Here's how the part is built. I have some questions about the finished solid (model axes, mm). Coordinates: 2 decimals unless noted, no trailing zeros. Order: outer loops, then holes, each group sorted by start corner. A loop starts at its lowest first (then second) coordinate and runs counter-clockwise, first axis right, second up. Notation, with made-up numbers: M 23,73.5 L 48,73.5 A14 ccw 48,77.5 Z; hole C 15,68 d3. An arc over 180 degrees is marked long. Answer as CSV lines item,"result". Start each with the question number.
```python
from build123d import *

# Parameters (mm, degrees)
SKETCH1_W                 = 58
SKETCH1_H                 = 68
BOSS_EXTRUDE1_DEPTH       = 3
F_6_0MM_DOWEL_HOLE1_D     = 6
F_6_0MM_DOWEL_HOLE1_DEPTH = 3


with BuildPart() as part:
    # Sketch1 → Boss-Extrude1 (new body)
    with BuildSketch(Plane(origin=(0, 0, 0), x_dir=(1, 0, 0), z_dir=(0, 1, 0))):
        with Locations((2.631421053, -22.558871845)):
            Rectangle(SKETCH1_W, SKETCH1_H)
    extrude(amount=BOSS_EXTRUDE1_DEPTH)

    # Ø6.0mm Dowel Hole1
    with Locations(Plane(origin=(0, 0, 0), x_dir=(-1, 0, 0), z_dir=(0, -1, 0))):
        with Locations((11.303876488, -0.981472803)):
            Hole(F_6_0MM_DOWEL_HOLE1_D / 2, depth=F_6_0MM_DOWEL_HOLE1_DEPTH)


solid = part.part
```
1) I need wall thicknesses on line 1 (X direction, y = 1.45, z = 3.5); line 2 (X direction, y = 2.55, z = 2); line 3 (Z direction, x = -10.5, y = 2.4). Which ranges of each line are inside material? Lowest first, please. Write a range as [from, to].
2) If we mould it in two halves opening along Z, with no side actions, what happens to faces 1 (the face through (-13.68, 1.52, 2.81)), 2 (the face through (2, 1, 56.559)), 3 (the face through (-26.369, 1, 23))? For each: released by +Z, released by -Z, zero draft, split by the parting line, or undercut.
3) Suppose I cut it at A-A on x = -13. Please give me the cut outline in (y, z).
Output:
1,line 1,"[-26.37, -12.93], [-9.67, 31.63]"
1,line 2,"[-26.37, -14.13], [-8.48, 31.63]"
1,line 3,"[-11.44, -1.91], [3.87, 56.56]"
2,face 1,"undercut"
2,face 2,"released by +Z"
2,face 3,"zero draft"
3,outline,"M 0,-11.44 L 3,-11.44 L 3,-1.49 L 0,-1.49 Z; M 0,3.46 L 3,3.46 L 3,56.56 L 0,56.56 Z"
